Can you work these out from the model? Positions are in its coordinate system, mm. Face numbers are marked on the shaded views. A direction names the side the tool comes from. Coordinates: 2 decimals unless noted, no trailing zeros. Write each loop counter-clockwise with the first axis right and the second up, starting at its lowest first coordinate (ties: lowest second). Pieces come first, ordered by that corner, then holes. Notation, with made-up numbers: (27, 67) -> (32, 67) arc R20 ccw to (32, 92) -> close; hole circle Ø5 at (-34, 63.5). An arc over 180 degrees is marked (long way). Use one line per item in the form item = value.
```python
from build123d import *

# Parameters (mm, degrees)
F0_W      = 150
F0_H      = 100
F1_DEPTH  = 600
F2_W      = 150
F2_H      = 100
F3_DEPTH  = 600.001
F4_W      = 150
F4_H      = 100
F5_DEPTH  = 600.001
F6_R      = 50
F7_R      = 50
F9_DEPTH  = 60
F11_DEPTH = 60
F12_W     = 700
F12_H     = 300
F13_DEPTH = 600.001
F14_R     = 50
F15_R     = 50
F16_W     = 550
F16_H     = 480
F17_DEPTH = 50
F18_DEPTH = 25
F19_DEPTH = 250.001


with BuildPart() as f1:
    # F0 (on Front) → F1 (new body)
    with BuildSketch(Plane.XZ):
        with Locations((-775, -75)):
            Rectangle(F0_W, F0_H)
        Polygon((-700, -25), (-700, -125), (850, -125), (850, 125), (-850, 125), (-850, -25), align=None)
    extrude(amount=F1_DEPTH)

    # F2 (on face) → F3 (cut, through all)
    with BuildSketch(Plane.XZ.offset(600)):
        with Locations((-775, -75)):
            Rectangle(F2_W, F2_H)
    extrude(amount=-F3_DEPTH, mode=Mode.SUBTRACT)

    # F4 (on face) → F5 (cut, through all)
    with BuildSketch(Plane.XZ.offset(600)):
        with Locations((775, -75)):
            Rectangle(F4_W, F4_H)
    extrude(amount=-F5_DEPTH, mode=Mode.SUBTRACT)

    # F6
    f6_edges = [f1.edges().sort_by_distance(p)[0] for p in [
        (-700, -300, -25),
    ]]
    fillet(f6_edges, radius=F6_R)

    # F7
    f7_edges = [f1.edges().sort_by_distance(p)[0] for p in [
        (700, -300, -25),
    ]]
    fillet(f7_edges, radius=F7_R)

    # F8 (on face) → F9 (join)
    with BuildSketch(Plane(origin=(0, 0, 0), x_dir=(-1, 0, 0), z_dir=(0, 1, 0))):
        with BuildLine():
            Line((-850, 125), (850, 125))
            ThreePointArc((850, 125), (0, 389.079291), (-850, 125))
        make_face()
    extrude(amount=-F9_DEPTH)

    # F10 (on face) → F11 (join)
    with BuildSketch(Plane.XZ.offset(600)):
        with BuildLine():
            Line((850, -25), (850, 125))
            ThreePointArc((850, 125), (0, 389.079291), (-850, 125))
            Line((-850, 125), (-850, -25))
            Line((-850, -25), (-750, -25))
            ThreePointArc((-750, -25), (-714.644661, -39.644661), (-700, -75))
            Line((-700, -75), (-700, -125))
            Line((-700, -125), (700, -125))
            Line((700, -125), (700, -75))
            ThreePointArc((700, -75), (714.644661, -39.644661), (750, -25))
            Line((750, -25), (850, -25))
        make_face()
    extrude(amount=-F11_DEPTH)

    # F12 (on face) → F13 (cut, through all)
    with BuildSketch(Plane.XZ.offset(600)):
        with Locations((0, -125)):
            Rectangle(F12_W, F12_H)
    extrude(amount=-F13_DEPTH, mode=Mode.SUBTRACT)

    # F14
    f14_edges = [f1.edges().sort_by_distance(p)[0] for p in [
        (350, -300, 25),
    ]]
    fillet(f14_edges, radius=F14_R)

    # F15
    f15_edges = [f1.edges().sort_by_distance(p)[0] for p in [
        (-350, -300, 25),
    ]]
    fillet(f15_edges, radius=F15_R)

    # F16 (on face) → F17 (join)
    with BuildSketch(Plane.XY.offset(125)):
        with Locations((0, -300)):
            Rectangle(F16_W, F16_H)
        with BuildLine():
            Line((100, -400), (-100, -400))
            ThreePointArc((-100, -400), (-200, -300), (-100, -200))
            Line((-100, -200), (100, -200))
            ThreePointArc((100, -200), (170.710678, -229.289322), (200, -300))
            ThreePointArc((200, -300), (170.710678, -370.710678), (100, -400))
        make_face(mode=Mode.SUBTRACT)
    extrude(amount=F17_DEPTH)

    # F16 (on face) → F18 (join)
    with BuildSketch(Plane.XY.offset(125)):
        with Locations((0, -300)):
            Rectangle(F16_W, F16_H)
        with BuildLine():
            Line((100, -400), (-100, -400))
            ThreePointArc((-100, -400), (-200, -300), (-100, -200))
            Line((-100, -200), (100, -200))
            ThreePointArc((100, -200), (170.710678, -229.289322), (200, -300))
            ThreePointArc((200, -300), (170.710678, -370.710678), (100, -400))
        make_face(mode=Mode.SUBTRACT)
    extrude(amount=F18_DEPTH)

    # F17_face (on face) → F19 (cut, through all)
    with BuildSketch(Plane(origin=(0, -300, 125), x_dir=(1, 0, 0), z_dir=(0, 0, 1))):
        with BuildLine():
            Line((100, 100), (-100, 100))
            ThreePointArc((-100, 100), (-200, 0), (-100, -100))
            Line((-100, -100), (100, -100))
            ThreePointArc((100, -100), (200, 0), (100, 100))
        make_face()
    extrude(amount=-F19_DEPTH, mode=Mode.SUBTRACT)


solid = f1.part
```
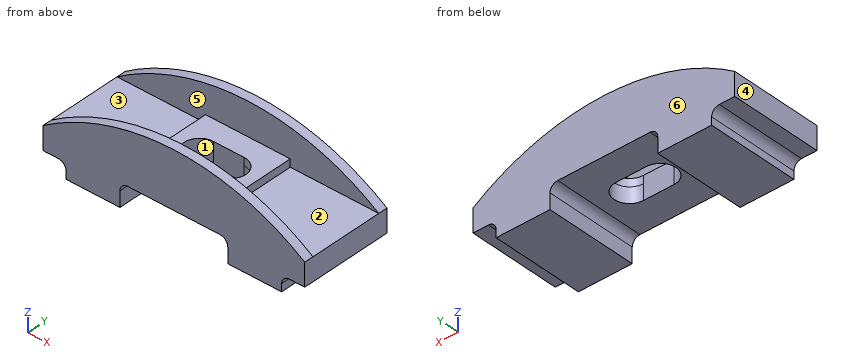
Q1. Suppose I cut it at C-C (x = -656). Write out the boundary of the cut face in (y, z), then the cut area to 3 significant figures.
Return value:
outline = (-600, -125) -> (0, -125) -> (0, 238.03) -> (-60, 238.03) -> (-60, 125) -> (-540, 125) -> (-540, 238.03) -> (-600, 238.03) -> close
area = 164,000 mm2
Q2. Suppose I cut it at B-B (z = 309). Write out the boundary of the cut face in (x, y), then the cut area to 3 significant figures.
Return value:
outline = (-483.55, -600) -> (483.55, -600) -> (483.55, -540) -> (-483.55, -540) -> close; (-483.55, -60) -> (483.55, -60) -> (483.55, 0) -> (-483.55, 0) -> close
area = 116,000 mm2
Q3. Thinking about a two-plate mould opening in Y: for the marked faces 4, 5 and 6, which applies, released by +Y, released by -Y, zero draft, split by the parting line, or undercut?
Return value:
face_4 = zero draft
face_5 = undercut
face_6 = released by +Y
Q4. For the marked faces 1, 2 and 3, which set-ups out of +Z, -Z, +X, -X, +Y, -Y let a thin tool reach every point of the face, with its end or its side?
Return value:
face_1 = +Z, -Z
face_2 = +Z, +X
face_3 = +Z, -X
Q5. If I drill on line 1 (Y direction, x = 19.5, z = 328); line 2 (X direction, y = -396.5, z = -95.5); line 3 (Y direction, x = -67.5, z = 102), over which ranges is the centre line in solid material (lowest first)? Write a range as from..to.
Return value:
line_1 = -600..-540, -60..0
line_2 = -700..-350, 350..700
line_3 = -600..-400, -200..0
Q6. Suppose I cut it at D-D (z = 191.5). Write out the boundary of the cut face in (x, y).
Return value:
outline = (-744.11, -600) -> (744.11, -600) -> (744.11, -540) -> (-744.11, -540) -> close; (-744.11, -60) -> (744.11, -60) -> (744.11, 0) -> (-744.11, 0) -> close
Q7. Will these pins go through, and if not, where does the flat tip stop? pin 1 (1.5 mm diameter, centred on x = 436.5, y = -407.5, fed in from +Z); pin 2 (12 mm diameter, centred on x = 139, z = 186, fed in from +Y).
Return value:
pin_1 = 125
pin_2 = 0
Q8. Suppose I cut it at A-A (z = 51). Write out the boundary of the cut face in (x, y), then the cut area to 3 significant figures.
Return value:
outline = (-850, -600) -> (850, -600) -> (850, 0) -> (-850, 0) -> close; hole (-100, -400) -> (100, -400) arc R100 ccw to (100, -200) -> (-100, -200) arc R100 ccw to start
area = 949,000 mm2
